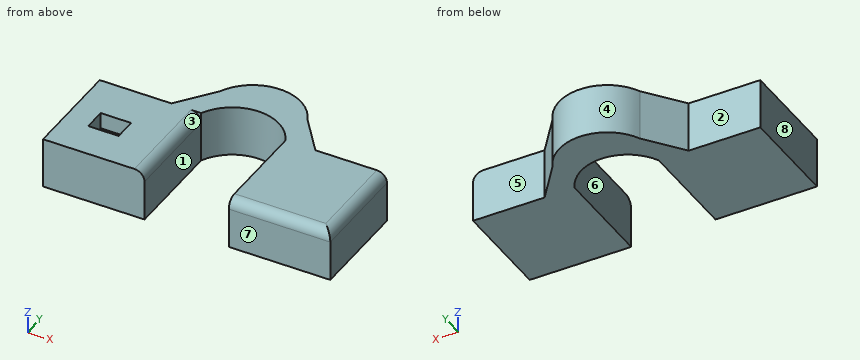
```python
from build123d import *

# Parameters (mm, degrees)
F0_W     = 50
F0_H     = 25
F1_DEPTH = 50
F2_R     = 5
F2_2_R   = 5
F3_W     = 15
F3_H     = 11
F3_R     = 5
F4_DEPTH = 8
F7_DEPTH = 25


with BuildPart() as f1:
    # F0 (on Front) → F1 (new body)
    with BuildSketch(Plane.XZ):
        with Locations((51.8986206502, 45.4651199281)):
            Rectangle(F0_W, F0_H)
    extrude(amount=F1_DEPTH)

    # F2
    f2_edges = [f1.edges().sort_by_distance(p)[0] for p in [
        (76.898621, -25, 57.96512),
    ]]
    fillet(f2_edges, radius=F2_R)

    # F3 (on face) → F4 (cut)
    with BuildSketch(Plane.XY.offset(57.9651199281)):
        with Locations((46.6270151734, -26.549421221)):
            Rectangle(F3_W, F3_H)
        with Locations((140.8739293367, -25.6193820387)):
            Circle(F3_R)
    extrude(amount=-F4_DEPTH, mode=Mode.SUBTRACT)



with BuildPart() as f1b:
    # F0 (on Front) → F1, piece 2 (new body)
    with BuildSketch(Plane.XZ):
        with Locations((143.3739293367, 45.4651199281)):
            Rectangle(F0_W, F0_H)
    extrude(amount=F1_DEPTH)

    # F2#2
    f2_2_edges = [f1b.edges().sort_by_distance(p)[0] for p in [
        (168.373929, -25, 57.96512),
        (143.373929, -50, 57.96512),
    ]]
    fillet(f2_2_edges, radius=F2_2_R)


with BuildPart() as f1_1:
    add(f1.part)

    add(f1b.part)  # F7 merges F1b
    # F6 (on offset) → F7 (join)
    with BuildSketch(Plane(origin=(0, 0, 32.9651199281), x_dir=(1, 0, 0), z_dir=(0, 0, -1))):
        with BuildLine():
            ThreePointArc((118.3739293367, 0), (97.6362749934, -13.1297755552), (76.8986206502, 0))
            Line((76.8986206502, 0), (62.1641688049, 0))
            Line((62.1641688049, 0), (76.054610312, -17.9887413979))
            ThreePointArc((76.054610312, -17.9887413979), (97.6362749934, -31.8841869417), (119.2179396749, -17.9887413979))
            Line((119.2179396749, -17.9887413979), (133.108381182, 0))
            Line((133.108381182, 0), (118.3739293367, 0))
        make_face()
    extrude(amount=-F7_DEPTH)


solid = f1_1.part
```
Here's how the part is built. I have some questions about the finished solid (model axes, mm). Face numbers are marked on the shaded views. A direction names the side the tool comes from. Give positions to 0.01 mm unless a question says otherwise; leave off trailing zeros. Loops run counter-clockwise (first coordinate to the right, second up) from the corner with the lowest first, then second, coordinate; pieces in that order, holes last. Notation, with made-up numbers: M 83.25,86 L 106.25,86 A15 cw 106.25,100 Z; hole C -36.75,-7 d3. An arc over 180 degrees is marked long. Use one line per item in the form item = value. Start each with the question number.
Q1. If we section it at D-D (y = -5): Write out the boundary of the cut face in (x, z), then the cut area to 3 significant figures.
Q2. Which directions (+Z, -Z, +X, -X, +Y, -Y) give clear straight access to the entire face, cutting with the end or side of a thin tool? Please do the marked faces 1, 2, 3, 4 and 5.
Q3. If we section it at B-B (z = 47.5): Write out the boundary of the cut face in (x, y).
Q4. If we section it at A-A (y = -30): Write out the boundary of the cut face in (x, z), then the cut area to 3 significant figures.
Q5. If we section it at C-C (x = 57.5): Write out the boundary of the cut face in (y, z).
Q6. I need wall thicknesses on line 1 along X through (y, z) = (-33, 36.75); line 2 along X through (y, z) = (2, 57.25); line 3 along Y through (x, z) = (139, 43.5). Which ranges of each line are inside material? Lowest first, please.
Q7. Will these pins go through, and if not, where does the flat tip stop? pin 1 Ø2.5 at (x, z) = (44, 52) entering from +Y; pin 2 Ø3 at (x, z) = (114, 42) entering from +Y; pin 3 Ø5.5 at (x, y) = (50, -27) entering from +Z.
Q8. Thinking about a two-plate mould opening in X: for the marked faces 6, 7 and 8, which applies, +X half, -X half, draft (parallel to the pull), parting line (faces both ways), or undercut?
Taken from the geometry:
q1.outline = M 26.9,32.97 L 76.9,32.97 L 76.9,52.97 A5 ccw 71.9,57.97 L 26.9,57.97 Z; M 118.37,32.97 L 168.37,32.97 L 168.37,52.97 A5 ccw 163.37,57.97 L 118.37,57.97 Z
q1.area = 2,490 mm^2
q2.face_1 = +Z, -Z, -Y
q2.face_2 = +Z, -Z, -X, +Y
q2.face_3 = +Z, -Y
q2.face_4 = +Z, -Z, +Y
q2.face_5 = +Z, -Z, +X, +Y
q3.outline = M 26.9,-50 L 76.9,-50 L 76.9,0 A22.94 cw 118.37,0 L 118.37,-50 L 168.37,-50 L 168.37,0 L 133.11,0 L 119.22,17.99 A23.71 ccw 76.05,17.99 L 62.16,0 L 26.9,0 Z
q4.outline = M 26.9,32.97 L 76.9,32.97 L 76.9,52.97 A5 ccw 71.9,57.97 L 54.13,57.97 L 54.13,49.97 L 39.13,49.97 L 39.13,57.97 L 26.9,57.97 Z; M 118.37,32.97 L 168.37,32.97 L 168.37,52.97 A5 ccw 163.37,57.97 L 118.37,57.97 Z
q4.area = 2,370 mm^2
q5.outline = M -50,32.97 L 0,32.97 L 0,57.97 L -50,57.97 Z
q6.line_1 = 26.9 to 76.9, 118.37 to 168.37
q6.line_2 = 63.71 to 77.97, 117.3 to 131.56
q6.line_3 = -50 to 0
q7.pin_1 = 0
q7.pin_2 = 26.65
q7.pin_3 = 49.97
q8.face_6 = undercut
q8.face_7 = draft
q8.face_8 = -X half
